```python
from build123d import *

# Parameters (mm, degrees)
ESQUISSE1_W             = 433.5
ESQUISSE1_H             = 1837
BOSS_EXTRU_1_DEPTH      = 10
BOSS_EXTRU_2_DEPTH      = 25
BOSS_EXTRU_2_DEPTH_BACK = 40
ESQUISSE2_W             = 72
ESQUISSE2_H             = 72


with BuildPart() as part:
    # Esquisse1 → Boss.-Extru.1 (new body)
    with BuildSketch(Plane.XY):
        Rectangle(ESQUISSE1_W, ESQUISSE1_H)
    extrude(amount=BOSS_EXTRU_1_DEPTH)

    # Esquisse2 → Boss.-Extru.2 (add, two sides: drawn at the far end of the back side and taken through both)
    with BuildSketch(Plane.XY.offset(10).offset(-BOSS_EXTRU_2_DEPTH_BACK)):
        with Locations((-150.75, -36)):
            Rectangle(ESQUISSE2_W, ESQUISSE2_H)
    extrude(amount=BOSS_EXTRU_2_DEPTH + BOSS_EXTRU_2_DEPTH_BACK)


solid = part.part
```
Geometry check sheet. Reference: the model listing, model coordinates, mm. A direction names the side the tool comes from. Round coordinates to 2 decimals unless told otherwise and drop trailing zeros. Order: outer loops, then holes, each group sorted by start corner. A loop starts at its lowest first (then second) coordinate and runs counter-clockwise, first axis right, second up. Notation, with made-up numbers: (55.5, -39) - (102.5, -39) arc R16 cw to (102.5, -35) - close; hole circle Ø4 at (79, -19). An arc over 180 degrees is marked (long way). Use a Markdown table: item, result. Add a question column.
1) Gauge pin test, flat ends, axial feed: P1, Ø3, axis at x = -11.5, y = 481, coming from the +Z side; P2, Ø7.5, axis at x = -143.5, z = 17.5, coming from the +Y side; P3, Ø2, axis at x = -8.5, y = 580.5, coming from the -Z side; P4, Ø2, axis at y = 521, z = -2.5, coming from the -X side. Record the tip position at first contact, or that the pin passes through.
2) Set-up check for faces 4 (the flat face through (-151, -35, -30)), 5 (the flat face through (-114.75, -37, -15)), 6 (the flat face through (-186.75, -37, -15)): record each of +Z, -Z, +X, -X, +Y, -Y from which the full face is reachable in a straight line by a thin tool's end or side.
3) Section check B-B (y = 786). Record the cut outline in (x, z).
4) Thickness scan on line 1 along Y through (x, z) = (-143.5, -7); line 2 along Z through (x, y) = (-24.5, -136). Record the ranges inside material, lowest first.
5) Mould release check, pull along Y, two halves, no side actions. Record for faces 1 (the flat face through (-151, 0, -15)), 2 (the flat face through (-151, -72, -15)), 3 (the flat face through (-3, 13, 10)): released by +Y, released by -Y, zero draft, split by the parting line, or undercut.
6) Section check C-C (x = 20). Record the cut outline in (y, z).
7) Section check A-A (x = -150.5). Record the cut outline in (y, z).
Established:
| question | item | result |
|---|---|---|
| 1 | P1 | z = 10 |
| 1 | P2 | y = 0 |
| 1 | P3 | z = 0 |
| 1 | P4 | through |
| 2 | face 4 | -Z, +X, -X, +Y, -Y |
| 2 | face 5 | -Z, +X, +Y, -Y |
| 2 | face 6 | -Z, -X, +Y, -Y |
| 3 | outline | (-216.75, 0) - (216.75, 0) - (216.75, 10) - (-216.75, 10) - close |
| 4 | line 1 | -72 to 0 |
| 4 | line 2 | 0 to 10 |
| 5 | face 1 | released by +Y |
| 5 | face 2 | released by -Y |
| 5 | face 3 | zero draft |
| 6 | outline | (-918.5, 0) - (918.5, 0) - (918.5, 10) - (-918.5, 10) - close |
| 7 | outline | (-918.5, 0) - (-72, 0) - (-72, -30) - (0, -30) - (0, 0) - (918.5, 0) - (918.5, 10) - (0, 10) - (0, 35) - (-72, 35) - (-72, 10) - (-918.5, 10) - close |
